from build123d import *

# Parameters (mm, degrees)
SKETCH1_W           = 143
SKETCH1_H           = 31
BOSS_EXTRUDE1_DEPTH = 1.6
SKETCH2_W           = 23.8
SKETCH2_H           = 13.7
BOSS_EXTRUDE2_DEPTH = 8
SKETCH3_W           = 50.8
SKETCH3_H           = 25.4
BOSS_EXTRUDE3_DEPTH = 10.2


with BuildPart() as part:
    # Sketch1 → Boss-Extrude1 (new body)
    with BuildSketch(Plane(origin=(0, 0, 0), x_dir=(1, 0, 0), z_dir=(0, 1, 0))):
        Rectangle(SKETCH1_W, SKETCH1_H)
    extrude(amount=BOSS_EXTRUDE1_DEPTH)

    # Sketch2 → Boss-Extrude2 (add)
    with BuildSketch(Plane(origin=(0, 1.6, 0), x_dir=(1, 0, 0), z_dir=(0, 1, 0))):
        with Locations((45, 0)):
            Rectangle(SKETCH2_W, SKETCH2_H)
    extrude(amount=BOSS_EXTRUDE2_DEPTH)

    # Sketch3 → Boss-Extrude3 (add)
    with BuildSketch(Plane(origin=(0, 1.6, 0), x_dir=(1, 0, 0), z_dir=(0, 1, 0))):
        with Locations((-35, 0)):
            Rectangle(SKETCH3_W, SKETCH3_H)
    extrude(amount=BOSS_EXTRUDE3_DEPTH)


solid = part.part
Check sheet for the modelled part. Datum: model origin and axes. Units: mm. A direction names the side the tool comes from. Round coordinates to 2 decimals unless told otherwise and drop trailing zeros. Order: outer loops, then holes, each group sorted by start corner. A loop starts at its lowest first (then second) coordinate and runs counter-clockwise, first axis right, second up.
(1) Cross-section at C-C, the plane x = 39.5. Enter the section's corners in (y, z).
(2) Cross-section at A-A, the plane y = 5. Enter the section's corners in (x, z).
(3) Cross-section at B-B, the plane z = 5. Enter the section's corners in (x, y).
(4) Go/stop test with flat-tipped pins: P1, Ø1.5, axis at y = 4.5, z = 7.5, coming from the +X side; P2, Ø1.5, axis at x = -9, y = 4, coming from the +Z side; P3, Ø7, axis at x = 49.5, z = 1.5, coming from the +Y side. Record where each tip stops, or that it passes through.
(5) Cross-section at D-D, the plane z = 10.5. Enter the section's corners in (x, y), and give its area (3 significant figures).
(6) Draft check along X on faces 1 (the flat face through (56.9, 6, 0)), 2 (the flat face through (15, 1.6, 0)), 3 (the flat face through (45, 6, -6.85)). Enter one of: pulls with the +X half, pulls with the -X half, needs draft (parallel to the pull), parting line crosses it, or undercut.
(7) Scan lines: probe 1 along X at (y, z) = (8.75, -5.5); probe 2 along Z at (x, y) = (-55, 10); probe 3 along Y at (x, z) = (50, -2). Record each from-to range of solid material in increasing order.
(8) Access from +Z, -Z, +X, -X, +Y, -Y to the whole of each face (thin tool, end or side, straight path). Record for faces 4 (the flat face through (45, 6, 6.85)), 5 (the flat face through (-35, 7, -12.7)), 6 (the flat face through (45, 9.6, 0)), 7 (the flat face through (-9.6, 7, 0)).
Check sheet entries:
1. outline: (0, -15.5) - (1.6, -15.5) - (1.6, -6.85) - (9.6, -6.85) - (9.6, 6.85) - (1.6, 6.85) - (1.6, 15.5) - (0, 15.5) - close
2. outline: (-60.4, -12.7) - (-9.6, -12.7) - (-9.6, 12.7) - (-60.4, 12.7) - close; (33.1, -6.85) - (56.9, -6.85) - (56.9, 6.85) - (33.1, 6.85) - close
3. outline: (-71.5, 0) - (71.5, 0) - (71.5, 1.6) - (56.9, 1.6) - (56.9, 9.6) - (33.1, 9.6) - (33.1, 1.6) - (-9.6, 1.6) - (-9.6, 11.8) - (-60.4, 11.8) - (-60.4, 1.6) - (-71.5, 1.6) - close
4. P1: stops at x = 56.9
4. P2: stops at z = 12.7
4. P3: stops at y = 9.6
5. outline: (-71.5, 0) - (71.5, 0) - (71.5, 1.6) - (-9.6, 1.6) - (-9.6, 11.8) - (-60.4, 11.8) - (-60.4, 1.6) - (-71.5, 1.6) - close
5. area: 747 mm2
6. face 1: pulls with the +X half
6. face 2: undercut
6. face 3: needs draft
7. probe 1: x = -60.4 to -9.6, 33.1 to 56.9
7. probe 2: z = -12.7 to 12.7
7. probe 3: y = 0 to 9.6
8. face 4: +Z, +X, +Y
8. face 5: -Z, +X, -X, +Y
8. face 6: +Z, -Z, +X, +Y
8. face 7: +Z, -Z, +Y
